Autodesk Inventor part; units mm, degrees
ref_plane "YZ Plane" through (0, 0, 0) normal (1, 0, 0) x (0, 1, 0)
ref_plane "XZ Plane" through (0, 0, 0) normal (0, 1, 0) x (-1, 0, 0)
ref_plane "XY Plane" through (0, 0, 0) normal (0, 0, 1) x (1, 0, 0)
sketch "Sketch1" plane through (0, 0, 0) normal (0, 1, 0) x (-1, 0, 0)
  line L0 (-60.452, -60.452) -> (60.452, -60.452)
  line L1 (60.452, -60.452) -> (60.452, 60.452)
  line L2 (60.452, 60.452) -> (-60.452, 60.452)
  line L3 (-60.452, 60.452) -> (-60.452, -60.452)
  line L4 (-60.452, -60.452) -> (60.452, 60.452) construction
  line L5 (60.452, -60.452) -> (-60.452, 60.452) construction
  point P0 (0, 0)
  dimension "d0" = 120.904
  dimension "d1" = 120.904
extrude "Extrusion1" add sketch "Sketch1" along normal blind 2.54
sketch "Sketch2" plane through (0, 2.54, 0) normal (0, 1, 0) x (1, 0, 0)
  line L0 (60.452, 60.452) -> (-60.452, 60.452)
  line L1 (60.452, -60.452) -> (-60.452, -60.452)
  line L2 (-60.452, -60.452) -> (-60.452, 60.452)
  line L3 (-60.452, 60.452) -> (60.452, 60.452)
  line L4 (60.452, 60.452) -> (60.452, -60.452)
  line L5 (60.452, -60.452) -> (-60.452, 60.452) construction
  line L6 (-60.452, -60.452) -> (60.452, 60.452) construction
  line L7 (59.182, -59.182) -> (-59.182, -59.182)
  line L8 (-59.182, -59.182) -> (-59.182, 59.182)
  line L9 (-59.182, 59.182) -> (59.182, 59.182)
  line L10 (59.182, 59.182) -> (59.182, -59.182)
  line L11 (59.182, -59.182) -> (-59.182, 59.182) construction
  line L12 (-59.182, -59.182) -> (59.182, 59.182) construction
  point P0 (0, 0)
  dimension "d4" = 118.364
  dimension "d5" = 118.364
extrude "Extrusion2" add sketch "Sketch2" along normal blind 82.804
sketch "Sketch3" plane through (0, 2.54, 0) normal (0, 1, 0) x (1, 0, 0)
  circle A0 centre (0, -25.4) radius 2.0828
  circle A1 centre (0, 25.4) radius 2.0828
  point P0 (0, 0)
  dimension "d10" = 4.1656
  dimension "d11" = 4.1656
extrude "Extrusion3" cut sketch "Sketch3" against normal through all
sketch "Sketch4" plane through (0, 2.54, 0) normal (0, 1, 0) x (1, 0, 0)
  line L0 (32.9946, -9.9949) -> (-32.9946, 9.9949) construction
  line L1 (-32.9946, -9.9949) -> (32.9946, 9.9949) construction
  circle A0 centre (-32.9946, -9.9949) radius 1.4986
  circle A1 centre (-32.9946, 9.9949) radius 1.4986
  circle A2 centre (32.9946, -9.9949) radius 1.4986
  circle A3 centre (32.9946, 9.9949) radius 1.4986
  line L2 (50, -50) -> (-50, 50) construction
  line L3 (-50, -50) -> (50, 50) construction
  circle A4 centre (43.65, -42.38) radius 1.4224
  circle A5 centre (43.65, 42.38) radius 1.4224
  circle A6 centre (-42.38, 42.38) radius 1.4224
  circle A7 centre (-42.38, -42.38) radius 1.4224
  point P0 (0, 0)
  dimension "d14" = 65.9892
  dimension "d15" = 19.9898
  dimension "d16" = 2.9972
  dimension "d17" = 2.9972
  dimension "d18" = 2.9972
  dimension "d19" = 2.9972
  dimension "d20" = 100
  dimension "d21" = 100
  dimension "d28" = 2.8448
  dimension "d29" = 2.8448
  dimension "d30" = 2.8448
  dimension "d31" = 2.8448
extrude "Extrusion4" cut sketch "Sketch4" against normal through all
sketch "Sketch5" plane through (-59.182, 2.54, 59.182) normal (1, 0, 0) x (0, 0, -1)
  line L0 (0, 0) -> (0, 82.804)
  circle A0 centre (59.182, 19.05) radius 3.175
  point P0 (59.182, -2.54)
  dimension "d34" = 6.35
extrude "Extrusion5" cut sketch "Sketch5" against normal through all
sketch "Sketch7" plane through (59.182, 2.54, -59.182) normal (-1, 0, 0) x (0, 0, 1)
  line L0 (0, 0) -> (0, 82.804)
  line L1 (0, 19.05) -> (9.1821, 19.05) construction
  circle A0 centre (25.454, 19.05) radius 3.175
  circle A1 centre (58.7915, 19.05) radius 3.175
  circle A2 centre (88.1602, 19.05) radius 3.175
  point P0 (59.182, -2.54)
  dimension "d50" = 6.35
  dimension "d51" = 6.35
  dimension "d52" = 6.35
extrude "Extrusion6" cut sketch "Sketch7" against normal through all
properties part number "546-1550Z137-Combiner"
Read the model definition and answer for the solid it produces. Units are mm, in the model's axes. A direction names the side the tool comes from. Round coordinates to 2 decimals unless told otherwise and drop trailing zeros. Order: outer loops, then holes, each group sorted by start corner. A loop starts at its lowest first (then second) coordinate and runs counter-clockwise, first axis right, second up.
1) The part is cut by section A-A on y = 21.59. Write down the section's boundary in (x, z) (1 decimal).
2) For faces 1 (the face through (1, 43, 59.182)), 2 (the face through (0.96, 1.29, -23.55)), 3 (the face through (-59.81, 24.74, 0.41)), 4 (the face through (60.452, 42, 1)), 5 (the face through (59.8, 23.7, -36.1)), determine the directions among +Z, -Z, +X, -X, +Y, -Y from which every point of the face is accessible in a straight line to the end or side of a thin tool.
3) The part is cut by section B-B on z = -25.4. Write down the section's boundary in (x, y), plus the area to 3 significant figures.
4) The part is cut by section D-D on y = 71. Write down the section's boundary in (x, z), plus the area to 3 significant figures.
5) The mould has two halves that part along Y. Classify faces 6 (the face through (59.182, 43, -1)), 7 (the face through (59.808, 24.738, 28.565)), 8 (the face through (1, 0, 1)), 9 (the face through (1, 2.54, 1)): released by +Y, released by -Y, zero draft, split by the parting line, or undercut.
6) The part is cut by section C-C on x = 0. Write down the section's boundary in (y, z).
7) Straight lines are drawn through the part: L1, parallel to X at y = 0.9, z = 42.38; L2, parallel to Z at x = 0, y = 2.05; L3, parallel to X at y = 42, z = -28.5. For each, find the intervals that lie inside material, in ascending order.
8) Flat-ended cylindrical pins translate along their axes: pin 1 (4 mm diameter, centred on x = -43.5, z = -10, fed in from +Y); pin 2 (5 mm diameter, centred on x = 32.99, z = -9.99, fed in from -Y); pin 3 (1.7 mm diameter, centred on x = 43.65, z = -42.38, fed in from -Y). Find the tip coordinate at first contact, or state that the pin passes through.
Resolved:
1. outline: (-60.5, -60.5) - (60.5, -60.5) - (60.5, -36.9) - (59.2, -36.9) - (59.2, -59.2) - (-59.2, -59.2) - (-59.2, -3.2) - (-60.5, -3.2) - close; (-60.5, 3.2) - (-59.2, 3.2) - (-59.2, 59.2) - (59.2, 59.2) - (59.2, 32.2) - (60.5, 32.2) - (60.5, 60.5) - (-60.5, 60.5) - close; (59.2, -30.6) - (60.5, -30.6) - (60.5, -3.6) - (59.2, -3.6) - close; (59.2, 2.8) - (60.5, 2.8) - (60.5, 25.8) - (59.2, 25.8) - close
2. face 1: +Y
2. face 2: +Y, -Y
2. face 3: -X
2. face 4: +Z, -Z, +X, +Y, -Y
2. face 5: +X
3. outline: (-60.45, 0) - (-2.08, 0) - (-2.08, 2.54) - (-59.18, 2.54) - (-59.18, 85.34) - (-60.45, 85.34) - close; (2.08, 0) - (60.45, 0) - (60.45, 85.34) - (59.18, 85.34) - (59.18, 2.54) - (2.08, 2.54) - close
3. area: 507 mm2
4. outline: (-60.45, -60.45) - (60.45, -60.45) - (60.45, 60.45) - (-60.45, 60.45) - close; hole (-59.18, -59.18) - (59.18, -59.18) - (59.18, 59.18) - (-59.18, 59.18) - close
4. area: 608 mm2
5. face 6: zero draft
5. face 7: undercut
5. face 8: released by -Y
5. face 9: released by +Y
6. outline: (0, -60.45) - (85.34, -60.45) - (85.34, -59.18) - (2.54, -59.18) - (2.54, -27.48) - (0, -27.48) - close; (0, -23.32) - (2.54, -23.32) - (2.54, 23.32) - (0, 23.32) - close; (0, 27.48) - (2.54, 27.48) - (2.54, 59.18) - (85.34, 59.18) - (85.34, 60.45) - (0, 60.45) - close
7. L1: x = -60.45 to -43.8, -40.96 to 42.23, 45.07 to 60.45
7. L2: z = -60.45 to -27.48, -23.32 to 23.32, 27.48 to 60.45
7. L3: x = -60.45 to -59.18, 59.18 to 60.45
8. pin 1: stops at y = 2.54
8. pin 2: stops at y = 0
8. pin 3: passes through
